from build123d import *

# Parameters (mm, degrees)
CROQUIS1_W              = 700
CROQUIS1_H              = 550
SALIENTE_EXTRUIR1_DEPTH = 3
CROQUIS2_W              = 25
CROQUIS2_H              = 75
CROQUIS2_W_2            = 104.094566175
CROQUIS2_H_2            = 25
SALIENTE_EXTRUIR2_DEPTH = 75
CROQUIS4_R              = 12.5
CORTAR_EXTRUIR1_DEPTH   = 570
CROQUIS5_R              = 12.5
CORTAR_EXTRUIR2_DEPTH   = 740
CROQUIS7_R              = 12.5
SALIENTE_EXTRUIR4_DEPTH = 500


with BuildPart() as part:
    # Croquis1 → Saliente-Extruir1 (new body)
    with BuildSketch(Plane.XY):
        Rectangle(CROQUIS1_W, CROQUIS1_H)
    extrude(amount=SALIENTE_EXTRUIR1_DEPTH)

    # Croquis2 → Saliente-Extruir2 (add)
    with BuildSketch(Plane.XY.offset(3)):
        Polygon((350, 275), (350, 200), (350, 175), (245.905433825, 175), (245.905433825, 275), align=None)
        with Locations((-337.5, 237.5)):
            Rectangle(CROQUIS2_W, CROQUIS2_H)
        with Locations((297.952716913, -262.5)):
            Rectangle(CROQUIS2_W_2, CROQUIS2_H_2)
    extrude(amount=SALIENTE_EXTRUIR2_DEPTH)

    # Croquis4 → Cortar-Extruir1 (cut)
    with BuildSketch(Plane.XZ.offset(275)):
        with Locations((297.952716912, 40.5)):
            Circle(CROQUIS4_R)
    extrude(amount=-CORTAR_EXTRUIR1_DEPTH, mode=Mode.SUBTRACT)

    # Croquis5 → Cortar-Extruir2 (cut)
    with BuildSketch(Plane(origin=(350, 0, 0), x_dir=(0, 0, -1), z_dir=(1, 0, 0))):
        with Locations(Location((-40.5, 225, 0), (0, 0, 90))):
            Circle(CROQUIS5_R)
    extrude(amount=-CORTAR_EXTRUIR2_DEPTH, mode=Mode.SUBTRACT)

    # Croquis7 → Saliente-Extruir4 (add)
    with BuildSketch(Plane.XY.offset(3)):
        with Locations((-325, 170)):
            Circle(CROQUIS7_R)
    extrude(amount=SALIENTE_EXTRUIR4_DEPTH)


solid = part.part
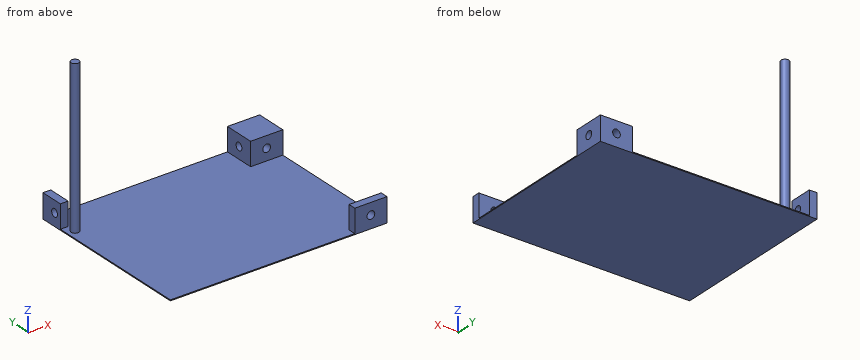
Design review of the part built by this model. Coordinates are the model's own, in mm. Round coordinates to 2 decimals unless told otherwise and drop trailing zeros. Loops run counter-clockwise (first coordinate to the right, second up) from the corner with the lowest first, then second, coordinate; pieces in that order, holes last. Notation, with made-up numbers: (3, 45) - (17, 45) arc R15 ccw to (17, 62) - close; hole circle Ø4 at (69, -18). An arc over 180 degrees is marked (long way). One line per item, written item: value. Start each with the question number.
1) Consider section C-C on x = -209.5. Give the boundary of the cut face in (y, z), then the cut area to 3 significant figures.
2) Consider section D-D on z = 441. Give the boundary of the cut face in (x, y), then the cut area to 3 significant figures.
3) Consider section B-B on y = 107. Give the boundary of the cut face in (x, z).
4) To check wall thickness, follow L1, parallel to X at y = 241.5, z = 40.5; L2, parallel to Y at x = 338, z = 40.5; L3, parallel to Z at x = -67.5, y = -157.5. State the ranges of each line that lie inside material, in increasing order. Write a range as from..to.
5) Insertion check: pin 1 Ø12.5 at (x, y) = (-335.5, 228.5) entering from +Z; pin 2 Ø20 at (x, z) = (-334.5, 23) entering from -Y; pin 3 Ø22.5 at (y, z) = (225, 40.5) entering from +X; pin 4 Ø10 at (x, y) = (-219, -59) entering from +Z. Each pin has a flat end and moves straight along its axis. Give the tip position at first contact, or say it passes through.
6) Consider section A-A on z = 40.5. Give the number of separate pieces and of enclosed holes in the cut face, then the cut area to 3 significant figures.
Reported:
1. outline: (-275, 0) - (275, 0) - (275, 3) - (-275, 3) - close
1. area: 1,650 mm^2
2. outline: circle Ø25 at (-325, 170)
2. area: 491 mm^2
3. outline: (-350, 0) - (350, 0) - (350, 3) - (-350, 3) - close
4. L1: x = -350..-325, 245.91..285.45, 310.45..350
4. L2: y = -275..-250, 175..212.5, 237.5..275
4. L3: z = 0..3
5. pin 1: stops at z = 78
5. pin 2: stops at y = 157.5
5. pin 3: passes through
5. pin 4: stops at z = 3
6. separate pieces: 9
6. enclosed holes: 0
6. area: 9,650 mm^2
